Source: three-view drawing plus pictorial views. Frame: mm from the lowest corner of the part. Give positions to 0.01 mm unless a question says otherwise; leave off trailing zeros. Order: outer loops, then holes, each group sorted by start corner. A loop starts at its lowest first (then second) coordinate and runs counter-clockwise, first axis right, second up. Notation, with made-up numbers: M 89.5,22.25 L 138.5,22.25 A14 cw 138.5,49.25 Z; hole C 85.5,86 d6. An arc over 180 degrees is marked long. Use CSV: the item, a comma, the result in double quotes. Start each with the question number.
Item 1: First-contact query: pin 1 (6 mm diameter, centred on x = 8, y = 15, fed in from -Z); pin 2 (5 mm diameter, centred on y = 19.5, z = 6.5, fed in from +X). Flat tips, straight axial feed; report the tip coordinate or a pass-through.
Item 2: Ray query, probe 1 along Y at (x, z) = (8, 6.5); probe 2 along X at (y, z) = (17, 3.25); probe 3 along Y at (x, z) = (7, 1.75). Return the intervals inside material, ascending. Write a range as from..to.
Item 3: Section query A-A on y = 15. Return loops of the section in (x, z).
Item 4: Pull-direction query (Y, two-part tool) for the marked faces 1, 2 and 3; classes: +Y half, -Y half, draft (parallel to the pull), parting line (faces both ways), or undercut.
Item 5: Section query D-D on x = 12.5. Return loops of the section in (y, z), and give its area (3 significant figures).
Item 6: Section query B-B on x = 8.25. Return loops of the section in (y, z).
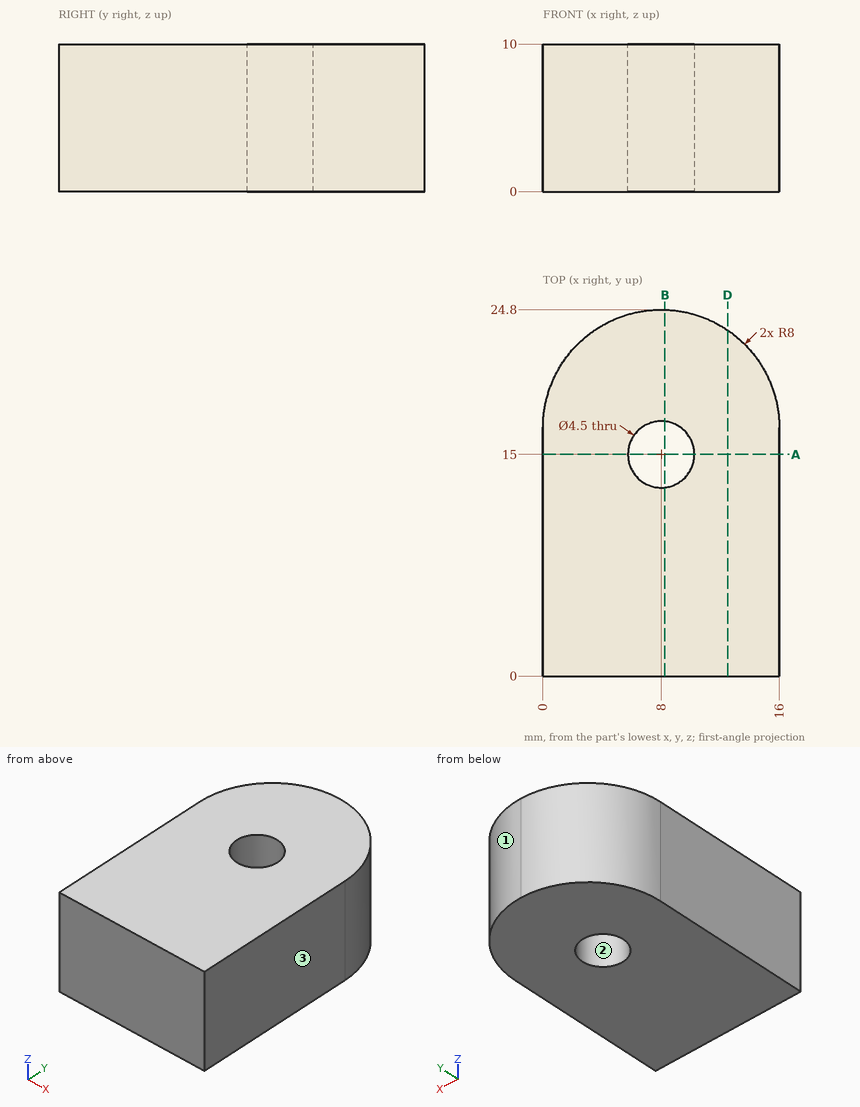
Verdict:
1,pin 1,"z = 0"
1,pin 2,"x = 16"
2,probe 1,"0..12.75, 17.25..24.8"
2,probe 2,"0..6.97, 9.03..16"
2,probe 3,"0..12.98, 17.02..24.74"
3,outline,"M 0,0 L 5.75,0 L 5.75,10 L 0,10 Z; M 10.25,0 L 16,0 L 16,10 L 10.25,10 Z"
4,face 1,"+Y half"
4,face 2,"undercut"
4,face 3,"draft"
5,outline,"M 0,0 L 23.41,0 L 23.41,10 L 0,10 Z"
5,area,"234 mm2"
6,outline,"M 0,0 L 12.76,0 L 12.76,10 L 0,10 Z; M 17.24,0 L 24.8,0 L 24.8,10 L 17.24,10 Z"
